from build123d import *

# Parameters (mm, degrees)
SKETCH1_R           = 7.875
BOSS_EXTRUDE1_DEPTH = 2
SKETCH1_3_R         = 10
BOSS_EXTRUDE2_DEPTH = 2
FILLET1_R           = 2
SKETCH2_R           = 5.875
CUT_EXTRUDE1_DEPTH  = 2


with BuildPart() as part:
    # Sketch1 → Boss-Extrude1 (new body)
    with BuildSketch(Plane(origin=(0, 0, 0), x_dir=(0, 0, -1), z_dir=(1, 0, 0))):
        Circle(SKETCH1_R)
    extrude(amount=BOSS_EXTRUDE1_DEPTH)

    # Sketch1<3> → Boss-Extrude2 (add)
    with BuildSketch(Plane(origin=(0, 0, 0), x_dir=(0, 0, -1), z_dir=(1, 0, 0))):
        Circle(SKETCH1_3_R)
    extrude(amount=-BOSS_EXTRUDE2_DEPTH)

    # Fillet1
    fillet1_edges = [part.edges().sort_by_distance(p)[0] for p in [
        (-2, 0, 10),
    ]]
    fillet(fillet1_edges, radius=FILLET1_R - 0.0001)  # a hair under: the kernel refuses the full size

    # Sketch2 → Cut-Extrude1 (cut)
    with BuildSketch(Plane(origin=(2, 0, 0), x_dir=(0, 0, -1), z_dir=(1, 0, 0))):
        Circle(SKETCH2_R)
    extrude(amount=-CUT_EXTRUDE1_DEPTH, mode=Mode.SUBTRACT)


solid = part.part
Source: CAD feature listing. Evaluate the final solid. Frame: model axes, mm. A direction names the side the tool comes from. Coordinates: 2 decimals unless noted, no trailing zeros. Order: outer loops, then holes, each group sorted by start corner. A loop starts at its lowest first (then second) coordinate and runs counter-clockwise, first axis right, second up.
Item 1: Cut plane C-C (x = 0.9). Return loops of the section in (y, z) (3 decimals).
Output values:
outline: circle Ø15.75 at (0, 0); hole circle Ø11.75 at (0, 0)
Item 2: Material intervals for line 1 (Y direction, x = 0.7, z = 0) (3 decimals); line 2 (X direction, y = -3, z = -4.5); line 3 (Z direction, x = 0.9, y = -3.5), sorted ascending.
Output values:
line 1: y = -7.875 to -5.875, 5.875 to 7.875
line 2: x = -2 to 0
line 3: z = -7.05 to -4.72, 4.72 to 7.05
Item 3: Pull-direction query (Z, two-part tool) for faces 3 (the face through (0, 0, 0)), 4 (the face through (1.014, 1.765, -5.604)), 5 (the face through (0.986, 7.808, 1.025)), 6 (the face through (-2, 0, 0)); classes: pulls with the +Z half, pulls with the -Z half, needs draft (parallel to the pull), parting line crosses it, or undercut.
Output values:
face 3: undercut
face 4: undercut
face 5: parting line crosses it
face 6: needs draft
Item 4: Set-up query: faces 1 (the face through (2, -1, 6)), 2 (the face through (0, -7, -4)). Return all of +Z, -Z, +X, -X, +Y, -Y with unobstructed straight access to the full face (end or side cutting, diameter ignored); none if empty.
Output values:
face 1: +Z, -Z, +X, +Y, -Y
face 2: +X
